```python
from build123d import *

# Parameters (mm, degrees)
F0_R     = 5
F1_DEPTH = 4
F2_R     = 5


with BuildPart() as f1:
    # F0 (on Top) → F1 (new body)
    with BuildSketch(Plane.XY):
        Polygon((0, 30), (0, 0), (220, 0), (230, 25.196342), (280, 25.196342), (280, 55.196342), (212.859735, 75), (195, 30), align=None)
        with Locations((15, 15)):
            Circle(F0_R, mode=Mode.SUBTRACT)
        with Locations((45, 15)):
            Circle(F0_R, mode=Mode.SUBTRACT)
        with Locations((211.182641, 37.196342)):
            Circle(F0_R, mode=Mode.SUBTRACT)
        with Locations((256.182641, 37.196342)):
            Circle(F0_R, mode=Mode.SUBTRACT)
        with Locations((217.044881, 59.405253)):
            Circle(F0_R, mode=Mode.SUBTRACT)
    extrude(amount=F1_DEPTH)

    # F2
    f2_edges = [f1.edges().sort_by_distance(p)[0] for p in [
        (0, 30, 2),
        (0, 0, 2),
        (220, 0, 2),
        (280, 25.196342, 2),
        (280, 55.196342, 2),
        (212.859735, 75, 2),
        (195, 30, 2),
        (230, 25.196342, 2),
    ]]
    fillet(f2_edges, radius=F2_R)


solid = f1.part
```
Geometry: final body of the model. Coordinates: model frame, mm. Round coordinates to 2 decimals unless told otherwise and drop trailing zeros. Order: outer loops, then holes, each group sorted by start corner. A loop starts at its lowest first (then second) coordinate and runs counter-clockwise, first axis right, second up. Notation, with made-up numbers: M -8,80 L 31,80 A5 cw 31,88 Z; hole C 11,-30 d2. An arc over 180 degrees is marked long. One line per item, written item: value.
(1) Cut plane A-A (x = 15). Return the cut outline in (y, z), and give its area (3 significant figures).
Result sheet:
outline: M 0,0 L 10,0 L 10,4 L 0,4 Z; M 20,0 L 30,0 L 30,4 L 20,4 Z
area: 80.0 mm2
(2) Cut plane C-C (z = 3.2). Return the cut outline in (x, y), and give its area (3 significant figures).
Result sheet:
outline: M 0,5 A5 ccw 5,0 L 216.61,0 A5 ccw 221.25,3.16 L 228.75,22.04 A5 cw 233.39,25.2 L 275,25.2 A5 ccw 280,30.2 L 280,51.46 A5 ccw 276.41,56.25 L 217.24,73.71 A5 ccw 211.18,70.76 L 196.25,33.16 A5 cw 191.61,30 L 5,30 A5 ccw 0,25 Z; hole C 15,15 d10; hole C 45,15 d10; hole C 211.18,37.2 d10; hole C 217.04,59.41 d10; hole C 256.18,37.2 d10
area: 9,360 mm2
(3) Cut plane D-D (x = 79). Return the cut outline in (y, z), and give its area (3 significant figures).
Result sheet:
outline: M 0,0 L 30,0 L 30,4 L 0,4 Z
area: 120 mm2
(4) Line query: probe 1 along Y at (x, z) = (45, 2.85); probe 2 along X at (y, z) = (40.5, 2.4); probe 3 along X at (y, z) = (12, 1.4). Output: solid intervals per line, ascending. Write a range as [from, to].
Result sheet:
probe 1: [0, 10], [20, 30]
probe 2: [199.17, 207.43], [214.94, 252.43], [259.94, 280]
probe 3: [0, 11], [19, 41], [49, 224.76]
(5) Cut plane B-B (y = 15). Return the cut outline in (x, z).
Result sheet:
outline: M 0,0 L 10,0 L 10,4 L 0,4 Z; M 20,0 L 40,0 L 40,4 L 20,4 Z; M 50,0 L 225.95,0 L 225.95,4 L 50,4 Z
(6) Pull-direction query (X, two-part tool) for faces 1 (the cylindrical face through (278.496, 26.622, 2.028)), 2 (the flat face through (203.82, 52.22, 1.97)), 3 (the cylindrical face through (17.307, 10.564, 1.972)); classes: pulls with the +X half, pulls with the -X half, needs draft (parallel to the pull), parting line crosses it, or undercut.
Result sheet:
face 1: pulls with the +X half
face 2: pulls with the -X half
face 3: undercut
(7) Pin query (flat end, axial travel): P1, Ø2, axis at y = 55, z = 1, coming from the -X side; P2, Ø1, axis at x = 172.5, z = 1.5, coming from the +Y side; P3, Ø1.5, axis at y = 56.5, z = 3, coming from the -X side. Return the tip coordinate at first contact, or that it passes through.
Result sheet:
P1: x = 204.53
P2: y = 30
P3: x = 205.22
